The model under review builds one solid part; all positions refer to its coordinate system, in mm. Face numbers are marked on the shaded views. A direction names the side the tool comes from. Coordinates: 2 decimals unless noted, no trailing zeros. Write each loop counter-clockwise with the first axis right and the second up, starting at its lowest first coordinate (ties: lowest second). Pieces come first, ordered by that corner, then holes. Notation, with made-up numbers: M 43,15 L 102,15 A24 ccw 102,54 Z; hole C 6,-2.5 d4. An arc over 180 degrees is marked long. Answer as a JSON object with one key per item and string values.
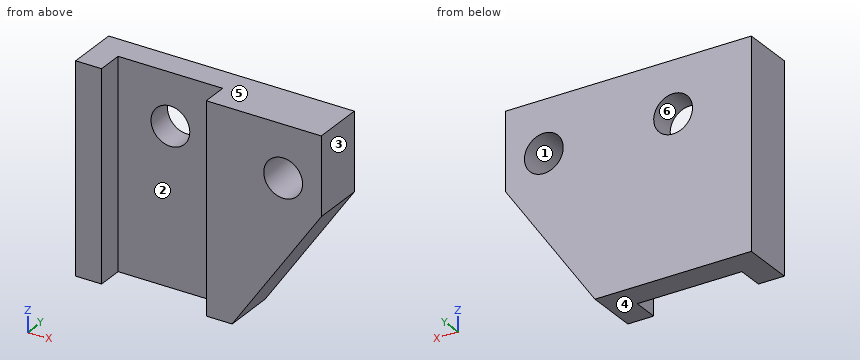
```python
from build123d import *

# Parameters (mm, degrees)
BOSS_EXTRU_1_DEPTH      = 16
ESQUISSE2_R             = 1.5
ENL_V_MAT_EXTRU_1_DEPTH = 26.159491251


with BuildPart() as part:
    # Esquisse1 → Boss.-Extru.1 (new body)
    with BuildSketch(Plane.XY):
        Polygon((10.1, -4), (19, -4), (19, 0), (0, 0), (0, -4), (2, -4), (2, -2), (10.1, -2), align=None)
    extrude(amount=BOSS_EXTRU_1_DEPTH)

    # Esquisse2 → Enlèv. mat.-Extru.1 (cut, through all)
    with BuildSketch(Plane(origin=(0, 0, 0), x_dir=(1, 0, 0), z_dir=(0, 1, 0))):
        with Locations(Location((6.05, -12, 0), (0, 0, 270))):
            Circle(ESQUISSE2_R)
        with Locations(Location((16.05, -12, 0), (0, 0, 270))):
            Circle(ESQUISSE2_R)
        Polygon((12.1, 0), (19, 0), (19, -10), align=None)
    extrude(amount=-ENL_V_MAT_EXTRU_1_DEPTH, mode=Mode.SUBTRACT)


solid = part.part
```
(1) Add section D-D on y = -1.1. Give the boundary of the cut face in (x, z), and give its area (3 significant figures).
Results list:
{"outline": "M 0,0 L 12.1,0 L 19,10 L 19,16 L 0,16 Z; hole C 6.05,12 d3; hole C 16.05,12 d3", "area": "255 mm²"}
(2) Draft analysis for pull direction Z (two halves, no side actions). For the marked faces 3, 4, 5 and 6, state which applies: released by +Z, released by -Z, zero draft, split by the parting line, or undercut.
Results list:
{"face 3": "zero draft", "face 4": "released by -Z", "face 5": "released by +Z", "face 6": "undercut"}
(3) For pin 1 Ø2.5 at (x, z) = (6.5, 8) entering from -Y; pin 2 Ø2 at (y, z) = (-3.5, 4) entering from +X, all flat-tipped, find the tip position at first contact; note any pin that passes through.
Results list:
{"pin 1": "y = -2", "pin 2": "x = 15.55"}
(4) Add section C-C on x = 6.05. Give the boundary of the cut face in (y, z), and give its area (3 significant figures).
Results list:
{"outline": "M -2,0 L 0,0 L 0,10.5 L -2,10.5 Z; M -2,13.5 L 0,13.5 L 0,16 L -2,16 Z", "area": "26.0 mm²"}
(5) Add section A-A on y = -2.55. Give the boundary of the cut face in (x, z), and give its area (3 significant figures).
Results list:
{"outline": "M 0,0 L 2,0 L 2,16 L 0,16 Z; M 10.1,0 L 12.1,0 L 19,10 L 19,16 L 10.1,16 Z; hole C 16.05,12 d3", "area": "133 mm²"}
(6) Wall thickness on line 1 along X through (y, z) = (-0.9, 12); line 2 along X through (y, z) = (-2.4, 12); line 3 along X through (y, z) = (-2.8, 15.25): over which ranges is each line inside the solid? List them lowest first. Write a range as from..to.
Results list:
{"line 1": "0..4.55, 7.55..14.55, 17.55..19", "line 2": "0..2, 10.1..14.55, 17.55..19", "line 3": "0..2, 10.1..19"}
(7) Add section B-B on z = 12. Give the boundary of the cut face in (x, y).
Results list:
{"outline": "M 0,-4 L 2,-4 L 2,-2 L 4.55,-2 L 4.55,0 L 0,0 Z; M 7.55,-2 L 10.1,-2 L 10.1,-4 L 14.55,-4 L 14.55,0 L 7.55,0 Z; M 17.55,-4 L 19,-4 L 19,0 L 17.55,0 Z"}
(8) For the marked faces 1 and 2, list the 3-axis set-ups (+Z, -Z, +X, -X, +Y, -Y) from which the entire face can be reached by the end or side of a thin tool; tool diameter is ignored.
Results list:
{"face 1": "+Y, -Y", "face 2": "+Z, -Z, -Y"}
